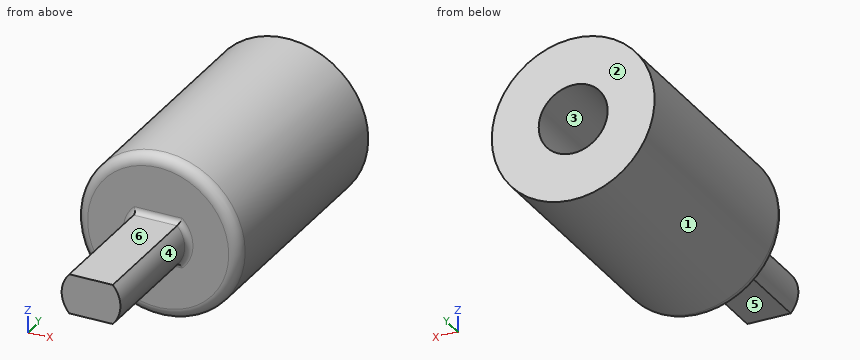
Solid Edge part; units mm, degrees
sketch "Sketch1" plane through (0, 0, 0) normal (0, -1, 0) x (1, 0, 0)
  circle A0 centre (0, 0) radius 3.175
  circle A1 centre (0, 0) radius 7.5
extrude "Protrusion1" add sketch "Sketch1" against normal blind 20
sketch "Sketch2" plane through (0, 0, 0) normal (0, -1, 0) x (1, 0, 0)
  circle A0 centre (0, 0) radius 7.5
extrude "ExtrudedProtrusion_2" add sketch "Sketch2" along normal blind 3
fillet "Round_1" radius 1 1 edges at (-7.5, -3, 0)
sketch "Sketch3" plane through (0, -3, 0) normal (0, -1, 0) x (1, 0, 0)
  line L0 (2.0018, -1.8183) -> (-2.0018, -1.8183)
  arc A0 (-2.0018, -1.8183) -> (-2.0018, 1.8183) centre (0, 0) cw
  line L1 (-2.0018, 1.8183) -> (2.0018, 1.8183)
  arc A1 (2.0018, 1.8183) -> (2.0018, -1.8183) centre (0, 0) cw
extrude "ExtrudedProtrusion_3" add sketch "Sketch3" along normal blind 12
fillet "Round_2" radius 0.5 5 edges at (0, -3, 1.8183) (2.7044, -3, 0) (0, -3, -1.8183) (-3.175, 0, 0) (-2.7044, -3, 0)
Check sheet for the modelled part. Datum: model origin and axes. Units: mm. Face numbers are marked on the shaded views. A direction names the side the tool comes from. Round coordinates to 2 decimals unless told otherwise and drop trailing zeros. Order: outer loops, then holes, each group sorted by start corner. A loop starts at its lowest first (then second) coordinate and runs counter-clockwise, first axis right, second up. Notation, with made-up numbers: (14, -35) - (23, -35) arc R23 cw to (23, -8) - close; hole circle Ø1 at (88, 24). An arc over 180 degrees is marked (long way). Answer as CSV lines item,"result". Start each with the question number.
1) Tool access check on the marked faces 4, 5 and 6. Record the directions out of +Z, -Z, +X, -X, +Y, -Y that give a thin tool (end or side, any length) a straight path to the whole face; none if there is none.
2) Depth check by flat-ended pin: pin 1 (4 mm diameter, centred on x = -6, y = 12.5, fed in from +Z); pin 2 (2.5 mm diameter, centred on x = 0.5, z = -1, fed in from +Y); pin 3 (1.5 mm diameter, centred on y = 16, z = 2, fed in from +X). Enter the tip coordinate at first touch or a pass-through.
3) Draft check along X on the marked faces 1, 2 and 3. Enter one of: +X half, -X half, draft (parallel to the pull), parting line (faces both ways), or undercut.
4) Scan lines: probe 1 along Z at (x, y) = (0, 15.5) (3 decimals); probe 2 along Y at (x, z) = (5.5, 0); probe 3 along Z at (x, y) = (2.5, 16). Record each from-to range of solid material in increasing order.
5) Section check A-A (x = 0). Record the cut outline in (y, z) (3 decimals).
6) Section check C-C (y = 11.5). Record the cut outline in (x, z) (3 decimals), then the cut area to 3 significant figures.
7) Section check B-B (z = 0). Record the cut outline in (x, y) (3 decimals), then the cut area to 3 significant figures.
Determined:
1,face 4,"+X, -Y"
1,face 5,"-Z, +X, -X, -Y"
1,face 6,"+Z, +X, -X, -Y"
2,pin 1,"z = 6.34"
2,pin 2,"y = 0"
2,pin 3,"x = 7.4"
3,face 1,"parting line"
3,face 2,"draft"
3,face 3,"undercut"
4,probe 1,"-7.5 to -3.175, 3.175 to 7.5"
4,probe 2,"-3 to 20"
4,probe 3,"-7.07 to -1.96, 1.96 to 7.07"
5,outline,"(-15, -1.818) - (-3.5, -1.818) arc R0.5 cw to (-3, -2.318) - (-3, -6.5) arc R1 ccw to (-2, -7.5) - (20, -7.5) - (20, -3.175) - (0.5, -3.175) arc R0.5 cw to (0, -2.675) - (0, 2.675) arc R0.5 cw to (0.5, 3.175) - (20, 3.175) - (20, 7.5) - (-2, 7.5) arc R1 ccw to (-3, 6.5) - (-3, 2.318) arc R0.5 cw to (-3.5, 1.818) - (-15, 1.818) - close"
6,outline,"circle Ø15 at (0, 0); hole circle Ø6.35 at (0, 0)"
6,area,"145 mm^2"
7,outline,"(-7.5, -2) arc R1 ccw to (-6.5, -3) - (-3.204, -3) arc R0.5 cw to (-2.704, -3.5) - (-2.704, -15) - (2.704, -15) - (2.704, -3.5) arc R0.5 cw to (3.204, -3) - (6.5, -3) arc R1 ccw to (7.5, -2) - (7.5, 20) - (3.175, 20) - (3.175, 0.5) arc R0.5 cw to (2.675, 0) - (-2.675, 0) arc R0.5 cw to (-3.175, 0.5) - (-3.175, 20) - (-7.5, 20) - close"
7,area,"283 mm^2"
